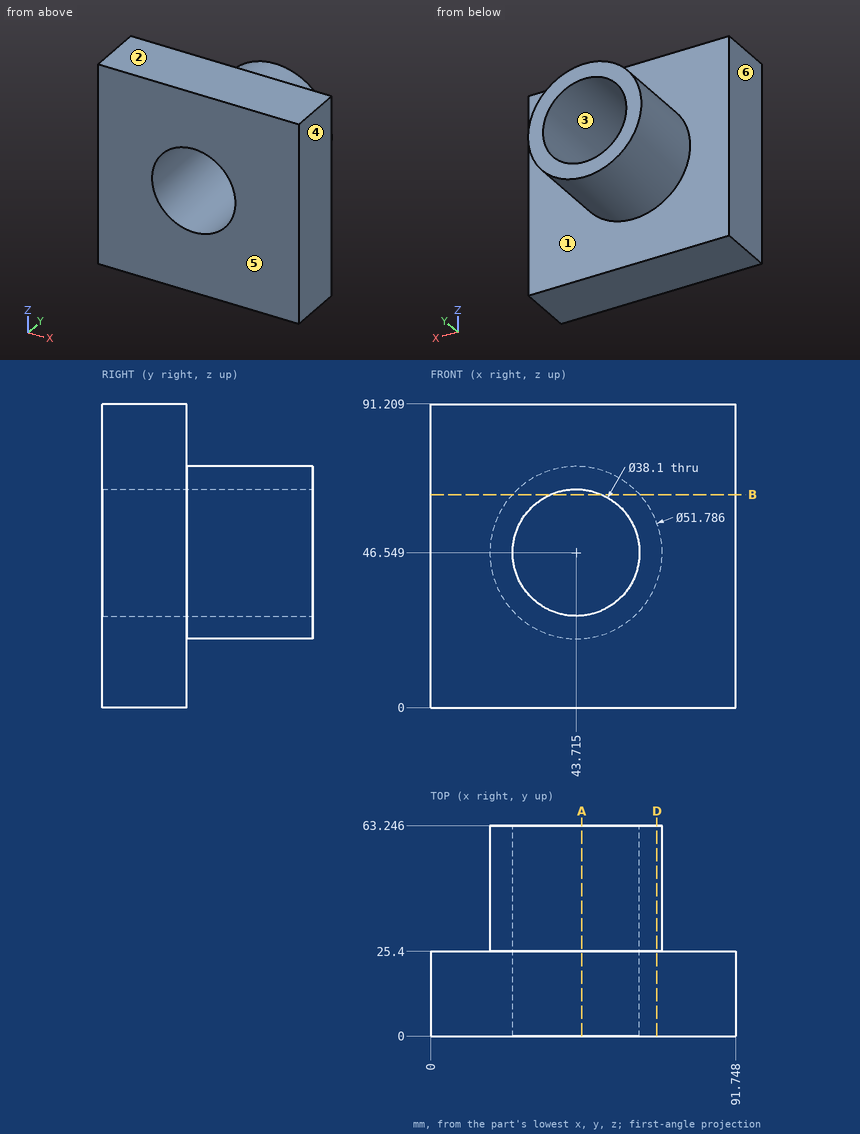
Source: three-view drawing plus pictorial views. Frame: mm from the lowest corner of the part. A direction names the side the tool comes from. Round coordinates to 2 decimals unless told otherwise and drop trailing zeros. Order: outer loops, then holes, each group sorted by start corner. A loop starts at its lowest first (then second) coordinate and runs counter-clockwise, first axis right, second up. Notation, with made-up numbers: (16, -8.5) - (75, -8.5) arc R14 ccw to (75, 8.5) - close; hole circle Ø3 at (-26, 33). An arc over 180 degrees is marked (long way). Answer in a Markdown table with one row per item.
Item 1: Section query B-B (z = 64). Return the cut outline in (x, y) (1 decimal), then the cut area to 3 significant figures.
Model answer:
| item | result |
|---|---|
| outline | (0, 0) - (36.1, 0) - (36.1, 63.2) - (24.6, 63.2) - (24.6, 25.4) - (0, 25.4) - close; (51.4, 0) - (91.7, 0) - (91.7, 25.4) - (62.8, 25.4) - (62.8, 63.2) - (51.4, 63.2) - close |
| area | 2,810 mm² |
Item 2: Section query A-A (x = 45.5). Return the cut outline in (y, z) (1 decimal), then the cut area to 3 significant figures.
Model answer:
| item | result |
|---|---|
| outline | (0, 0) - (25.4, 0) - (25.4, 20.7) - (63.2, 20.7) - (63.2, 27.6) - (0, 27.6) - close; (0, 65.5) - (63.2, 65.5) - (63.2, 72.4) - (25.4, 72.4) - (25.4, 91.2) - (0, 91.2) - close |
| area | 1,870 mm² |
Item 3: Mould query, pull axis X, two halves, no side actions, for the marked faces 3, 4, 5 and 6. Classes: released by +X, released by -X, zero draft, split by the parting line, or undercut.
Model answer:
| item | result |
|---|---|
| face 3 | undercut |
| face 4 | released by +X |
| face 5 | zero draft |
| face 6 | released by -X |
Item 4: Section query D-D (x = 68). Return the cut outline in (y, z) (1 decimal).
Model answer:
| item | result |
|---|---|
| outline | (0, 0) - (25.4, 0) - (25.4, 37.6) - (63.2, 37.6) - (63.2, 55.5) - (25.4, 55.5) - (25.4, 91.2) - (0, 91.2) - close |
Item 5: Line query: line 1 (Y direction, x = 40.5, z = 81.5); line 2 (Z direction, x = 47, y = 56) (1 decimal); line 3 (Z direction, x = 48, y = 50) (1 decimal). Output: solid intervals per line, ascending.
Model answer:
| item | result |
|---|---|
| line 1 | y = 0 to 25.4 |
| line 2 | z = 20.9 to 27.8, 65.3 to 72.2 |
| line 3 | z = 21 to 28, 65.1 to 72.1 |
Item 6: Reachability of the marked faces 1 and 2 from +Z, -Z, +X, -X, +Y, -Y: full face, straight path, thin tool, end or side. Return the list, or none.
Model answer:
| item | result |
|---|---|
| face 1 | +Y |
| face 2 | +Z, +X, -X, +Y, -Y |
Item 7: Pin query (flat end, axial travel): pin 1 (8 mm diameter, centred on x = 40.5, y = 50.5, fed in from +Z); pin 2 (2 mm diameter, centred on x = 39.5, y = 53, fed in from +Z); pin 3 (4 mm diameter, centred on x = 19.5, y = 49.5, fed in from +Z). Return the tip coordinate at first contact, or that it passes through.
Model answer:
| item | result |
|---|---|
| pin 1 | stops at z = 72.44 |
| pin 2 | stops at z = 72.24 |
| pin 3 | stops at z = 59.85 |
